Here's the drawing with two shaded views (mm, measured from the low corner). I have some questions. A direction names the side the tool comes from. Round coordinates to 2 decimals unless told otherwise and drop trailing zeros. Write each loop counter-clockwise with the first axis right and the second up, starting at its lowest first coordinate (ties: lowest second). Pieces come first, ordered by that corner, then holes.
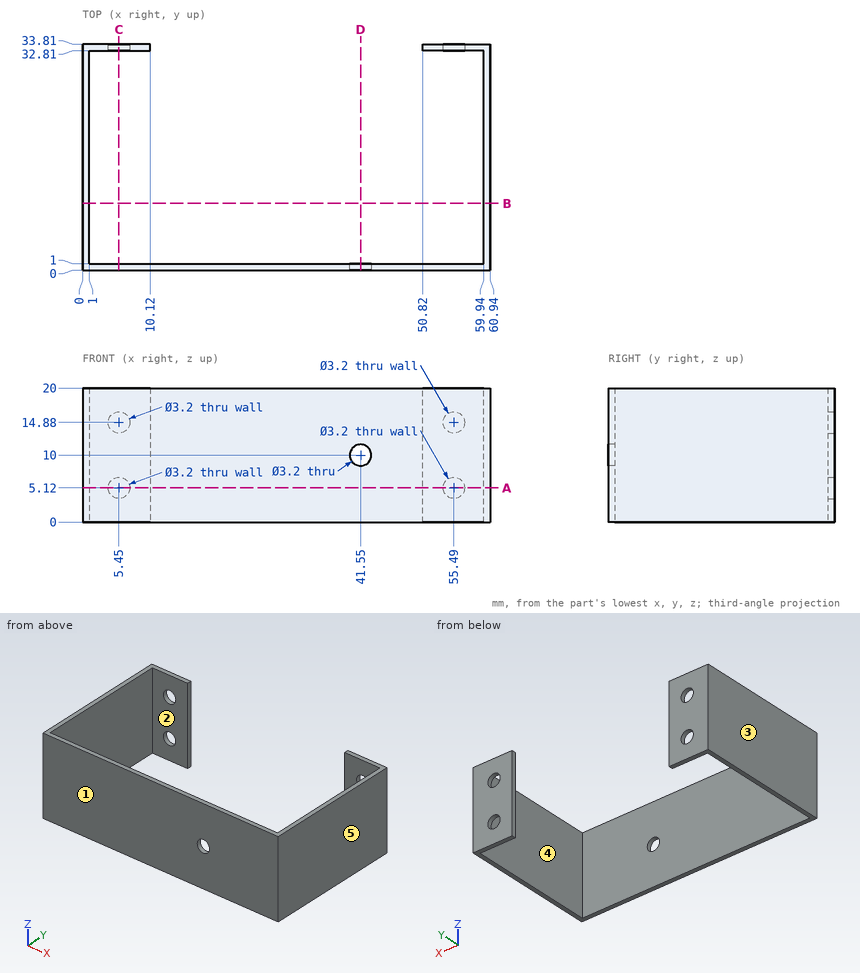
Q1. We'd pull the mould along X, two halves only. Please class the marked faces 1, 2 and 3: pulls with the +X half, pulls with the -X half, needs draft (parallel to the pull), parting line crosses it, or undercut.
Q2. Imagine slicing it at A-A, the plane z = 5.12. Write out the boundary of the cut face in (x, y).
Q3. If I drill on L1, parallel to Z at x = 55.49, y = 33; L2, parallel to X at y = 33.25, z = 14.88; L3, parallel to X at y = 22.5, z = 15, over which ranges is the centre line in solid material (lowest first)?
Q4. Imagine slicing it at C-C, the plane x = 5.45. Write out the boundary of the cut face in (y, z), then the cut area to 3 significant figures.
Q5. Imagine slicing it at D-D, the plane x = 41.55. Write out the boundary of the cut face in (y, z).
Q6. I'm going to push flat-ended pins straight in: pin 1 Ø1 at (x, z) = (19.5, 8) entering from -Y; pin 2 Ø1.9 at (x, z) = (5.45, 5.12) entering from +Y. Where does each tip first touch, or does it pass through?
Q7. Imagine slicing it at B-B, the plane y = 10. Write out the boundary of the cut face in (x, z).
Q8. On a 3-axis mill with a long thin cutter (end or side, diameter ignored), from which of +Z, -Z, +X, -X, +Y, -Y can I reach the whole of each face in a straight line? I mean the marked faces 4 and 5. Say none if no direction works.
Results found:
1. face 1: needs draft
1. face 2: undercut
1. face 3: pulls with the -X half
2. outline: (0, 0) - (60.94, 0) - (60.94, 33.81) - (57.09, 33.81) - (57.09, 32.81) - (59.94, 32.81) - (59.94, 1) - (1, 1) - (1, 32.81) - (3.85, 32.81) - (3.85, 33.81) - (0, 33.81) - close; (7.05, 32.81) - (10.12, 32.81) - (10.12, 33.81) - (7.05, 33.81) - close; (50.82, 32.81) - (53.89, 32.81) - (53.89, 33.81) - (50.82, 33.81) - close
3. L1: z = 0 to 3.52, 6.72 to 13.28, 16.48 to 20
3. L2: x = 0 to 3.85, 7.05 to 10.12, 50.82 to 53.89, 57.09 to 60.94
3. L3: x = 0 to 1, 59.94 to 60.94
4. outline: (0, 0) - (1, 0) - (1, 20) - (0, 20) - close; (32.81, 0) - (33.81, 0) - (33.81, 3.52) - (32.81, 3.52) - close; (32.81, 6.72) - (33.81, 6.72) - (33.81, 13.28) - (32.81, 13.28) - close; (32.81, 16.48) - (33.81, 16.48) - (33.81, 20) - (32.81, 20) - close
4. area: 33.6 mm2
5. outline: (0, 0) - (1, 0) - (1, 8.4) - (0, 8.4) - close; (0, 11.6) - (1, 11.6) - (1, 20) - (0, 20) - close
6. pin 1: stops at y = 0
6. pin 2: stops at y = 1
7. outline: (0, 0) - (1, 0) - (1, 20) - (0, 20) - close; (59.94, 0) - (60.94, 0) - (60.94, 20) - (59.94, 20) - close
8. face 4: +Z, -Z
8. face 5: +Z, -Z, +X, +Y, -Y
